Verification items for the finished model (mm, model axes). Face numbers are marked on the shaded views. A direction names the side the tool comes from. Coordinates: 2 decimals unless noted, no trailing zeros. Order: outer loops, then holes, each group sorted by start corner. A loop starts at its lowest first (then second) coordinate and runs counter-clockwise, first axis right, second up. Notation, with made-up numbers: M 65,48 L 110,48 A30 ccw 110,74 Z; hole C -3,10 d2. An arc over 180 degrees is marked long. Answer as a JSON object with one key per item and string values. Group by question number.
(1) Gauge pin test, flat ends, axial feed: pin 1 Ø5.5 at (x, y) = (0, 80) entering from -Z; pin 2 Ø1.5 at (x, y) = (-4.5, 31) entering from +Z. Record the tip position at first contact, or that the pin passes through.
(2) Material ranges on line 1 (Y direction, x = 4.85, z = 1.5); line 2 (Y direction, x = 4.75, z = 7); line 3 (Y direction, x = 1, z = -6), recorded low to high.
(3) Cross-section at A-A (y = 80). Enter the section's corners in (x, z), plus the area to 3 significant figures.
(4) Cross-section at C-C (y = 96). Enter the section's corners in (x, z), plus the area to 3 significant figures.
(5) Cross-section at B-B (x = 0). Enter the section's corners in (y, z).
(6) Access from +Z, -Z, +X, -X, +Y, -Y to the whole of each face (thin tool, end or side, straight path). Record for the marked faces 4 and 5.
(7) Cross-section at D-D (x = 6.5). Enter the section's corners in (y, z).
(8) Mould release check, pull along Y, two halves, no side actions. Record for the marked faces 1, 2 and 3: released by +Y, released by -Y, zero draft, split by the parting line, or undercut.
from build123d import *

# Parameters (mm, degrees)
SKIZZE1_W                       = 15
SKIZZE1_H                       = 15
AUFSATZ_LINEAR_AUSTRAGEN1_DEPTH = 4
SKIZZE2_W                       = 15
SKIZZE2_H                       = 5
AUFSATZ_LINEAR_AUSTRAGEN2_DEPTH = 96
SKIZZE3_W                       = 5
SKIZZE3_H                       = 10
AUFSATZ_LINEAR_AUSTRAGEN3_DEPTH = 10
SKIZZE4_R                       = 2.2
SCHNITT_LINEAR_AUSTRAGEN1_DEPTH = 5
SCHNITT_LINEAR_AUSTRAGEN2_REACH = 17
SKIZZE5_R                       = 2.2
SKIZZE6_R                       = 2.2
SCHNITT_LINEAR_AUSTRAGEN3_DEPTH = 16
SKIZZE7_R                       = 2.2
SCHNITT_LINEAR_AUSTRAGEN4_DEPTH = 6


with BuildPart() as part:
    # Skizze1 → Aufsatz-Linear austragen1 (new body)
    with BuildSketch(Plane(origin=(0, 0, 0), x_dir=(1, 0, 0), z_dir=(0, 1, 0))):
        Rectangle(SKIZZE1_W, SKIZZE1_H)
    extrude(amount=AUFSATZ_LINEAR_AUSTRAGEN1_DEPTH)

    # Skizze2 → Aufsatz-Linear austragen2 (add)
    with BuildSketch(Plane(origin=(0, 4, 0), x_dir=(1, 0, 0), z_dir=(0, 1, 0))):
        with Locations((0, 5)):
            Rectangle(SKIZZE2_W, SKIZZE2_H)
    extrude(amount=AUFSATZ_LINEAR_AUSTRAGEN2_DEPTH)

    # Skizze3 → Aufsatz-Linear austragen3 (add)
    with BuildSketch(Plane.XY.offset(-2.5)):
        with Locations((-5, 95)):
            Rectangle(SKIZZE3_W, SKIZZE3_H)
        with Locations((5, 95)):
            Rectangle(SKIZZE3_W, SKIZZE3_H)
    extrude(amount=AUFSATZ_LINEAR_AUSTRAGEN3_DEPTH)

    # Skizze4 → Schnitt-Linear austragen1 (cut, through all)
    with BuildSketch(Plane(origin=(0, 4, 0), x_dir=(1, 0, 0), z_dir=(0, 1, 0))):
        with Locations((0, -2.5)):
            Circle(SKIZZE4_R)
    extrude(amount=-SCHNITT_LINEAR_AUSTRAGEN1_DEPTH, mode=Mode.SUBTRACT)

    # Skizze5 → Schnitt-Linear austragen2 (cut, up to next)
    with BuildSketch(Plane(origin=(7.5, 0, 0), x_dir=(0, 0, -1), z_dir=(1, 0, 0)), mode=Mode.PRIVATE) as schnitt_linear_austragen2_sk1:
        with Locations((-1.5, 96)):
            Circle(SKIZZE5_R)
    schnitt_linear_austragen2_tool1 = extrude(schnitt_linear_austragen2_sk1.sketch, amount=-SCHNITT_LINEAR_AUSTRAGEN2_REACH, mode=Mode.PRIVATE) & part.part
    add(schnitt_linear_austragen2_tool1.solids().sort_by_distance((7.5, 96, 1.5))[0], mode=Mode.SUBTRACT)

    # Skizze6 → Schnitt-Linear austragen3 (cut, through all)
    with BuildSketch(Plane.ZY.offset(7.5)):
        with Locations((1.5, 96)):
            Circle(SKIZZE6_R)
    extrude(amount=-SCHNITT_LINEAR_AUSTRAGEN3_DEPTH, mode=Mode.SUBTRACT)

    # Skizze7 → Schnitt-Linear austragen4 (cut, through all)
    with BuildSketch(Plane.XY.offset(-2.5)):
        with Locations((0, 20)):
            Circle(SKIZZE7_R)
        with Locations((0, 80)):
            Circle(SKIZZE7_R)
    extrude(amount=-SCHNITT_LINEAR_AUSTRAGEN4_DEPTH, mode=Mode.SUBTRACT)


solid = part.part
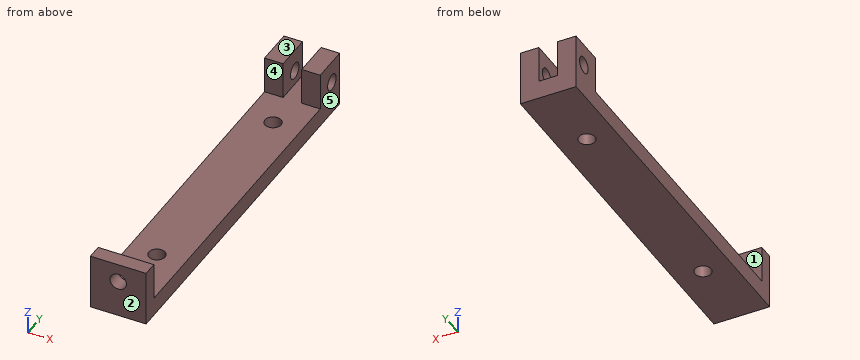
Taken from the geometry:
{
 "1": {"pin 1": "stops at z = -7.5", "pin 2": "stops at z = -2.5"},
 "2": {"line 1": "y = 0 to 4, 90 to 93.8, 98.2 to 100", "line 2": "y = 0 to 4, 90 to 100", "line 3": "y = 0 to 18.04, 21.96 to 78.04, 81.96 to 100"},
 "3": {"outline": "M -7.5,-7.5 L -2.2,-7.5 L -2.2,-2.5 L -7.5,-2.5 Z; M 2.2,-7.5 L 7.5,-7.5 L 7.5,-2.5 L 2.2,-2.5 Z", "area": "53.0 mm²"},
 "4": {"outline": "M -7.5,-7.5 L 7.5,-7.5 L 7.5,-0.7 L 2.5,-0.7 L 2.5,-2.5 L -2.5,-2.5 L -2.5,-0.7 L -7.5,-0.7 Z; M -7.5,3.7 L -2.5,3.7 L -2.5,7.5 L -7.5,7.5 Z; M 2.5,3.7 L 7.5,3.7 L 7.5,7.5 L 2.5,7.5 Z", "area": "131 mm²"},
 "5": {"outline": "M 0,-7.5 L 17.8,-7.5 L 17.8,-2.5 L 4,-2.5 L 4,0.3 L 0,0.3 Z; M 0,4.7 L 4,4.7 L 4,7.5 L 0,7.5 Z; M 22.2,-7.5 L 77.8,-7.5 L 77.8,-2.5 L 22.2,-2.5 Z; M 82.2,-7.5 L 100,-7.5 L 100,-2.5 L 82.2,-2.5 Z"},
 "6": {"face 4": "+Z, +X, -X", "face 5": "+Z, -Z, +X, +Y, -Y"},
 "7": {"outline": "M 0,-7.5 L 100,-7.5 L 100,7.5 L 90,7.5 L 90,-2.5 L 4,-2.5 L 4,7.5 L 0,7.5 Z; hole C 96,1.5 d4.4"},
 "8": {"face 1": "undercut", "face 2": "released by -Y", "face 3": "zero draft"}
}
